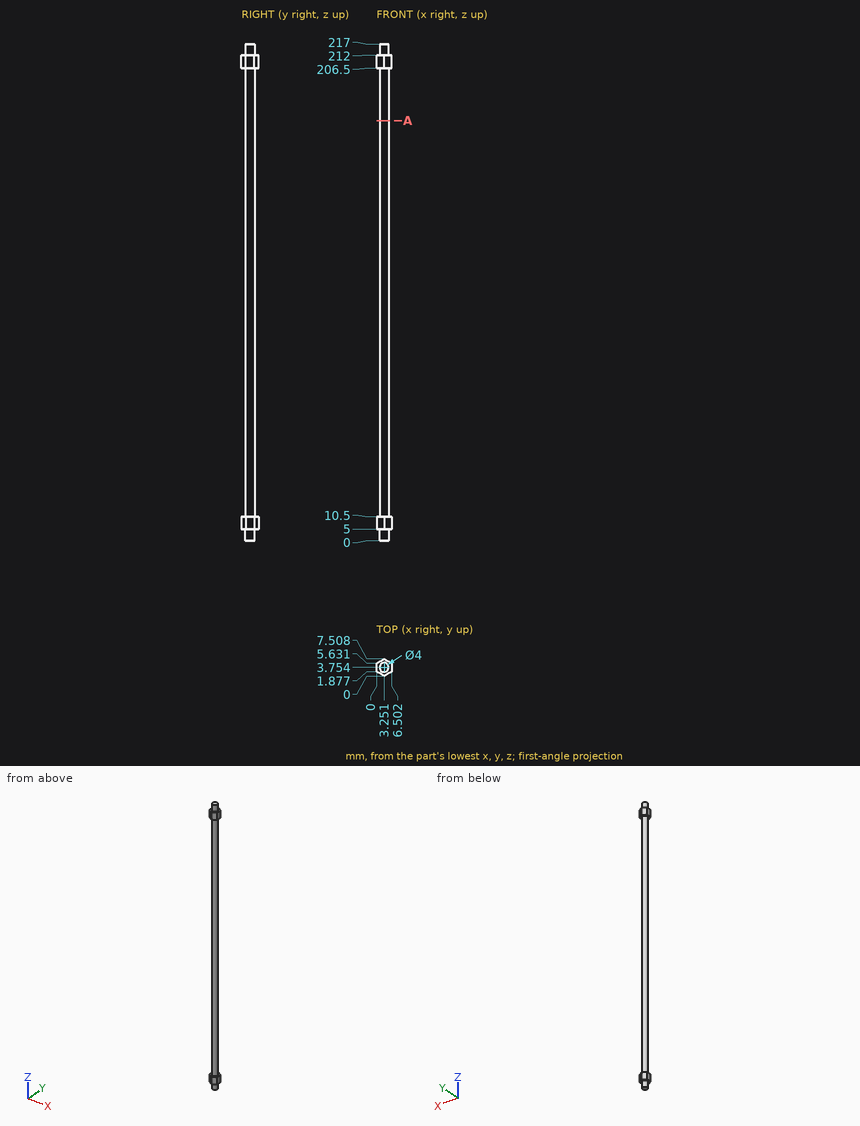
Input: dimensioned drawing with shaded views. Units: mm. Origin: part minimum x, y, z. Coordinates: 2 decimals unless noted, no trailing zeros. Loops run counter-clockwise (first coordinate to the right, second up) from the corner with the lowest first, then second, coordinate; pieces in that order, holes last. Notation, with made-up numbers: M -32,65 L 5,65 A28 cw 5,102 Z; hole C 37.5,34.5 d6. An arc over 180 degrees is marked long. One line per item, written item: value. Start each with the question number.
1) Pin query (flat end, axial travel): P1, Ø4, axis at y = 5, z = 79, coming from the +X side; P2, Ø1.5, axis at y = 3.5, z = 192, coming from the -X side. Return the tip coordinate at first contact, or that it passes through.
2) Material intervals for L1, parallel to Z at x = 0.75, y = 3.25; L2, parallel to X at y = 3.75, z = 29.5; L3, parallel to Y at x = 4.5, z = 111 (1 decimal), sorted ascending. Write a range as from..to.
3) Cut plane A-A (z = 183.5). Return loops of the section in (x, y), then the cut area to 3 significant figures.
Evaluation:
1. P1: x = 5.25
1. P2: x = 1.25
2. L1: 5..10.5, 206.5..212
2. L2: 1.25..5.25
2. L3: 2.2..5.3
3. outline: C 3.25,3.75 d4
3. area: 12.6 mm^2
